The listing builds one solid part. Answer for the finished solid, in the listing's coordinates (mm). A direction names the side the tool comes from. Round coordinates to 2 decimals unless told otherwise and drop trailing zeros. Write each loop counter-clockwise with the first axis right and the second up, starting at its lowest first coordinate (ties: lowest second). Pieces come first, ordered by that corner, then holes. Notation, with made-up numbers: (-39.75, 28) -> (-29.75, 28) arc R29 ccw to (-29.75, 64) -> close; hole circle Ø5 at (55, -6). An arc over 180 degrees is marked (long way). Write each question's results on one line, items separated by ' | '. Start each with the question number.
```python
from build123d import *

# Parameters (mm, degrees)
F0_W     = 500
F0_H     = 200
F0_R     = 3
F1_DEPTH = 30
F2_W     = 10
F2_H     = 10
F3_DEPTH = 500
F4_W     = 10
F4_H     = 1
F5_DEPTH = 500


with BuildPart() as f1:
    # F0 (on Right) → F1 (new body)
    with BuildSketch(Plane.YZ):
        Rectangle(F0_W, F0_H)
        with Locations((-235, -50)):
            Circle(F0_R, mode=Mode.SUBTRACT)
        with Locations((235, -50)):
            Circle(F0_R, mode=Mode.SUBTRACT)
        with Locations((-235, 0)):
            Circle(F0_R, mode=Mode.SUBTRACT)
        with Locations((-235, 50)):
            Circle(F0_R, mode=Mode.SUBTRACT)
        with Locations((235, 0)):
            Circle(F0_R, mode=Mode.SUBTRACT)
        with Locations((235, 50)):
            Circle(F0_R, mode=Mode.SUBTRACT)
    extrude(amount=F1_DEPTH)

    # F2 (on face) → F3 (join)
    with BuildSketch(Plane.XZ.offset(250)):
        with Locations((15, -105)):
            Rectangle(F2_W, F2_H)
    extrude(amount=-F3_DEPTH)

    # F4 (on face) → F5 (cut)
    with BuildSketch(Plane.XZ.offset(250)):
        with Locations((25, -94.5)):
            Rectangle(F4_W, F4_H)
    extrude(amount=-F5_DEPTH, mode=Mode.SUBTRACT)


solid = f1.part
```
Q1. The part is cut by section B-B, the plane x = 5.5. Write down the section's boundary in (y, z).
Q2. Each of these flat-tipped pins is pushed along its axis until it touches: pin 1 (3 mm diameter, centred on y = -34, z = -105.5, fed in from -X); pin 2 (2 mm diameter, centred on x = 3.5, y = 176.5, fed in from -Z); pin 3 (3 mm diameter, centred on y = 56, z = -103.5, fed in from +X); pin 4 (5 mm diameter, centred on y = 235, z = 0, fed in from -X). Where does it stop, or does it pass through?
Q3. The part is cut by section A-A, the plane y = -180. Write down the section's boundary in (x, z).
Q4. Find the intervals of material crossed by line 1 (Z direction, x = 13, y = -235); line 2 (Z direction, x = 21, y = 235); line 3 (Z direction, x = 20.5, y = 195.5), in increasing order.
Q5. For faces 1 (the flat face through (20, -4, -105)), 2 (the flat face through (15, -4, -110)), 3 (the flat face through (25, -4, -95)), 4 (the flat face through (5, -3, -100)), 5 (the flat face through (0, -3, 1)), determine the directions among +Z, -Z, +X, -X, +Y, -Y from which every point of the face is accessible in a straight line to the end or side of a thin tool.
Q6. Determine the mould class of faces 6 (the flat face through (25, -4, -94)), 7 (the flat face through (15, -250, -6)), 8 (the flat face through (15, -3, 100)) for opening direction Z: pulls with the +Z half, pulls with the -Z half, needs draft (parallel to the pull), parting line crosses it, or undercut.
Answers follow:
1) outline: (-250, -100) -> (250, -100) -> (250, 100) -> (-250, 100) -> close; hole circle Ø6 at (-235, -50); hole circle Ø6 at (-235, 0); hole circle Ø6 at (-235, 50); hole circle Ø6 at (235, -50); hole circle Ø6 at (235, 0); hole circle Ø6 at (235, 50)
2) pin 1: x = 10 | pin 2: z = -100 | pin 3: x = 20 | pin 4: through
3) outline: (0, -100) -> (10, -100) -> (10, -110) -> (20, -110) -> (20, -100) -> (30, -100) -> (30, -95) -> (20, -95) -> (20, -94) -> (30, -94) -> (30, 100) -> (0, 100) -> close
4) line 1: -110 to -53, -47 to -3, 3 to 47, 53 to 100 | line 2: -100 to -95, -94 to -53, -47 to -3, 3 to 47, 53 to 100 | line 3: -100 to -95, -94 to 100
5) face 1: -Z, +X, +Y, -Y | face 2: -Z, +X, -X, +Y, -Y | face 3: +X, +Y, -Y | face 4: -Z, -X, +Y, -Y | face 5: +Z, -Z, -X, +Y, -Y
6) face 6: undercut | face 7: needs draft | face 8: pulls with the +Z half
